from build123d import *

# Parameters (mm, degrees)
SKETCH_1_R          = 26.5
SKETCH_1_R_2        = 12.5
EXTRUDE_1_DEPTH     = 1
CUT_EXTRUDE_START   = 2.5
CUT_EXTRUDE_1_DEPTH = 1
SKETCH_3_R          = 1.52
CUT_EXTRUDE_2_DEPTH = 1


with BuildPart() as part:
    # 草图1 → 凸台-拉伸1 (new body)
    with BuildSketch(Plane.XY):
        Circle(SKETCH_1_R)
        Circle(SKETCH_1_R_2, mode=Mode.SUBTRACT)
    extrude(amount=EXTRUDE_1_DEPTH)

    # 草图2 → 切除-拉伸1 (cut)
    with BuildSketch(Plane(origin=(22.803986485, -9.350307143, -2.5), x_dir=(1, 0, 0), z_dir=(0, 0, 1)).offset(CUT_EXTRUDE_START)):
        with BuildLine():
            Line((-38.401990025, 19.652309401), (-42.257990025, 19.652309401))
            ThreePointArc((-42.257990025, 19.652309401), (-42.611543416, 19.505862792), (-42.757990025, 19.152309401))
            Line((-42.757990025, 19.152309401), (-42.757990025, 9.073309401))
            ThreePointArc((-42.757990025, 9.073309401), (-42.611543416, 8.719756011), (-42.257990025, 8.573309401))
            Line((-42.257990025, 8.573309401), (-38.401990025, 8.573309401))
            ThreePointArc((-38.401990025, 8.573309401), (-38.048436635, 8.719756011), (-37.901990025, 9.073309401))
            Line((-37.901990025, 9.073309401), (-37.901990025, 19.152309401))
            ThreePointArc((-37.901990025, 19.152309401), (-38.048436635, 19.505862792), (-38.401990025, 19.652309401))
        make_face()
        with BuildLine():
            Line((-8.221986913, 18.50930464), (-4.365986913, 18.50930464))
            ThreePointArc((-4.365986913, 18.50930464), (-4.012433522, 18.362858031), (-3.865986913, 18.00930464))
            Line((-3.865986913, 18.00930464), (-3.865986913, 6.02530464))
            ThreePointArc((-3.865986913, 6.02530464), (-4.012433522, 5.67175125), (-4.365986913, 5.52530464))
            Line((-4.365986913, 5.52530464), (-8.221986913, 5.52530464))
            ThreePointArc((-8.221986913, 5.52530464), (-8.575540303, 5.67175125), (-8.721986913, 6.02530464))
            Line((-8.721986913, 6.02530464), (-8.721986913, 18.00930464))
            ThreePointArc((-8.721986913, 18.00930464), (-8.575540303, 18.362858031), (-8.221986913, 18.50930464))
        make_face()
        with BuildLine():
            Line((-32.732983006, -4.858695665), (-14.351988011, -4.858695665))
            ThreePointArc((-14.351988011, -4.858695665), (-13.998434621, -5.005142274), (-13.851988011, -5.358695665))
            Line((-13.851988011, -5.358695665), (-13.851988011, -9.690695176))
            ThreePointArc((-13.851988011, -9.690695176), (-13.998434621, -10.044248567), (-14.351988011, -10.190695176))
            Line((-14.351988011, -10.190695176), (-32.732983006, -10.190695176))
            ThreePointArc((-32.732983006, -10.190695176), (-33.086536397, -10.044248567), (-33.232983006, -9.690695176))
            Line((-33.232983006, -9.690695176), (-33.232983006, -5.358695665))
            ThreePointArc((-33.232983006, -5.358695665), (-33.086536397, -5.005142274), (-32.732983006, -4.858695665))
        make_face()
        with BuildLine():
            Line((-35.099987523, 3.015306044), (-39.082987523, 3.015306044))
            ThreePointArc((-39.082987523, 3.015306044), (-39.436540913, 2.868859435), (-39.582987523, 2.515306044))
            Line((-39.582987523, 2.515306044), (-39.582987523, -3.499693956))
            ThreePointArc((-39.582987523, -3.499693956), (-39.436540913, -3.853247346), (-39.082987523, -3.999693956))
            Line((-39.082987523, -3.999693956), (-35.099987523, -3.999693956))
            ThreePointArc((-35.099987523, -3.999693956), (-34.746434132, -3.853247346), (-34.599987523, -3.499693956))
            Line((-34.599987523, -3.499693956), (-34.599987523, 2.515306044))
            ThreePointArc((-34.599987523, 2.515306044), (-34.746434132, 2.868859435), (-35.099987523, 3.015306044))
        make_face()
        with BuildLine():
            Line((-11.396988316, 3.142309279), (-7.921988316, 3.142309279))
            ThreePointArc((-7.921988316, 3.142309279), (-7.568434926, 2.99586267), (-7.421988316, 2.642309279))
            Line((-7.421988316, 2.642309279), (-7.421988316, -2.610690721))
            ThreePointArc((-7.421988316, -2.610690721), (-7.568434926, -2.964244111), (-7.921988316, -3.110690721))
            Line((-7.921988316, -3.110690721), (-11.396988316, -3.110690721))
            ThreePointArc((-11.396988316, -3.110690721), (-11.750541707, -2.964244111), (-11.896988316, -2.610690721))
            Line((-11.896988316, -2.610690721), (-11.896988316, 2.642309279))
            ThreePointArc((-11.896988316, 2.642309279), (-11.750541707, 2.99586267), (-11.396988316, 3.142309279))
        make_face()
    extrude(amount=CUT_EXTRUDE_1_DEPTH, mode=Mode.SUBTRACT)

    # 草图3 → 切除-拉伸2 (cut)
    with BuildSketch(Plane(origin=(22.803986485, -9.350307143, -2.5), x_dir=(1, 0, 0), z_dir=(0, 0, 1)).offset(CUT_EXTRUDE_START)):
        with Locations((-22.803986485, 32.400306763)):
            Circle(SKETCH_3_R)
        with Locations((-45.853986105, 9.350307143)):
            Circle(SKETCH_3_R)
        with Locations((-22.803986485, -13.699692477)):
            Circle(SKETCH_3_R)
        with Locations((0.246013135, 9.350307143)):
            Circle(SKETCH_3_R)
    extrude(amount=CUT_EXTRUDE_2_DEPTH, mode=Mode.SUBTRACT)


solid = part.part
Could you check a few things on this model? Use its own coordinates, in mm. Coordinates: 2 decimals unless noted, no trailing zeros. Order: outer loops, then holes, each group sorted by start corner. A loop starts at its lowest first (then second) coordinate and runs counter-clockwise, first axis right, second up. Notation, with made-up numbers: (67.25, -19.5) - (118.25, -19.5) arc R28 ccw to (118.25, 7.5) - close; hole circle Ø2 at (59, 70). An arc over 180 degrees is marked (long way). Answer in a Markdown table with one row per item. Add a question column.
(1) If we section it at B-B, the plane y = -23.05: Please give me the cut outline in (x, z), then the cut area to 3 significant figures.
(2) If we mould it in two halves opening along X, with no side actions, what happens to faces 1 (the face through (14.246, 22.345, 0.493)), 2 (the face through (11.4, 6.3, 0)), 3 (the face through (11.923, 3.755, 0.493))? For each: released by +X, released by -X, zero draft, split by the parting line, or undercut.
(3) If we section it at D-D, the plane x = -18.5: Please give me the cut outline in (y, z).
(4) I need wall thicknesses on L1, parallel to Y at x = 0, z = 0.5; L2, parallel to X at y = 10, z = 0.8; L3, parallel to Y at x = -1, z = 0.9. Which ranges of each line are inside material? Lowest first, please.
(5) If we section it at C-C, the plane x = 6: Please give me the cut outline in (y, z), then the cut area to 3 significant figures.
(6) Will these pins go through, and if not, where does the flat tip stop? pin 1 (0.5 mm diameter, centred on y = -16, z = 0.5, fed in from -X); pin 2 (0.5 mm diameter, centred on y = 3, z = 0.5, fed in from -X); pin 3 (6 mm diameter, centred on x = 10.5, y = -5.5, fed in from -Z); pin 4 (0.5 mm diameter, centred on x = 13, z = 0.5, fed in from +Y).
(7) If we section it at A-A, the plane x = 0: Please give me the cut outline in (y, z).
Results are:
| question | item | result |
|---|---|---|
| 1 | outline | (-13.07, 0) - (-1.52, 0) - (-1.52, 1) - (-13.07, 1) - close; (1.52, 0) - (13.07, 0) - (13.07, 1) - (1.52, 1) - close |
| 1 | area | 23.1 mm2 |
| 2 | face 1 | split by the parting line |
| 2 | face 2 | zero draft |
| 2 | face 3 | undercut |
| 3 | outline | (-18.97, 0) - (-0.78, 0) - (-0.78, 1) - (-18.97, 1) - close; (10.3, 0) - (18.97, 0) - (18.97, 1) - (10.3, 1) - close |
| 4 | L1 | y = -26.5 to -24.57, -21.53 to -19.54, -14.21 to -12.5, 12.5 to 21.53, 24.57 to 26.5 |
| 4 | L2 | x = -24.54 to -19.91, -15.14 to -7.5, 7.5 to 24.54 |
| 4 | L3 | y = -26.48 to -24.19, -21.91 to -19.54, -14.21 to -12.46, 12.46 to 21.91, 24.19 to 26.48 |
| 5 | outline | (-25.81, 0) - (-19.54, 0) - (-19.54, 1) - (-25.81, 1) - close; (-14.21, 0) - (-10.97, 0) - (-10.97, 1) - (-14.21, 1) - close; (10.97, 0) - (25.81, 0) - (25.81, 1) - (10.97, 1) - close |
| 5 | area | 24.4 mm2 |
| 6 | pin 1 | stops at x = -21.31 |
| 6 | pin 2 | stops at x = -26.36 |
| 6 | pin 3 | stops at z = 0 |
| 6 | pin 4 | stops at y = 23.23 |
| 7 | outline | (-26.5, 0) - (-24.57, 0) - (-24.57, 1) - (-26.5, 1) - close; (-21.53, 0) - (-19.54, 0) - (-19.54, 1) - (-21.53, 1) - close; (-14.21, 0) - (-12.5, 0) - (-12.5, 1) - (-14.21, 1) - close; (12.5, 0) - (21.53, 0) - (21.53, 1) - (12.5, 1) - close; (24.57, 0) - (26.5, 0) - (26.5, 1) - (24.57, 1) - close |
